The figure shows three views and two pictorial views of one solid part (mm, origin at its lowest corner). Answer the questions. A direction names the side the tool comes from. Round coordinates to 2 decimals unless told otherwise and drop trailing zeros. Order: outer loops, then holes, each group sorted by start corner. A loop starts at its lowest first (then second) coordinate and runs counter-clockwise, first axis right, second up. Notation, with made-up numbers: (85, 38.5) -> (116, 38.5) arc R17 cw to (116, 51.5) -> close; hole circle Ø6 at (80, 78.5). An arc over 180 degrees is marked (long way). Answer as a JSON object with one key per item and string values. Group by question number.
Item 1: Section B-B, the plane z = 38.1 is taken. Write down the section's boundary in (x, y).
Item 2: Section C-C, the plane y = 58.5 is taken. Write down the section's boundary in (x, z), plus the area to 3 significant figures.
Item 3: Consider probe 1 along Y at (x, z) = (6.25, 38.1); probe 2 along Z at (x, y) = (7, 38.1); probe 3 along Z at (x, y) = (11.25, 42.5) (1 decimal). Determine where each line is inside the solid, lowest interval first. Write a range as from..to.
Item 4: Section D-D, the plane z = 68.5 is taken. Write down the section's boundary in (x, y).
Item 5: For the marked faces 1 and 2, determine the directions among +Z, -Z, +X, -X, +Y, -Y from which every point of the face is accessible in a straight line to the end or side of a thin tool.
Item 6: Given P1, Ø3, axis at x = 4.5, y = 91, coming from the -Z side; P2, Ø2.5, axis at x = 8, y = 60.5, coming from the -Z side (1 decimal); P3, Ø4, axis at x = 10, z = 19.5, coming from the +Y side (1 decimal), each flat-ended and moving along its own axis, determine where each tip first touches the part or whether it passes through.
Item 7: The mould has two halves that part along Y. Classify the marked faces 3, 4 and 5: pulls with the +Y half, pulls with the -Y half, needs draft (parallel to the pull), parting line crosses it, or undercut.
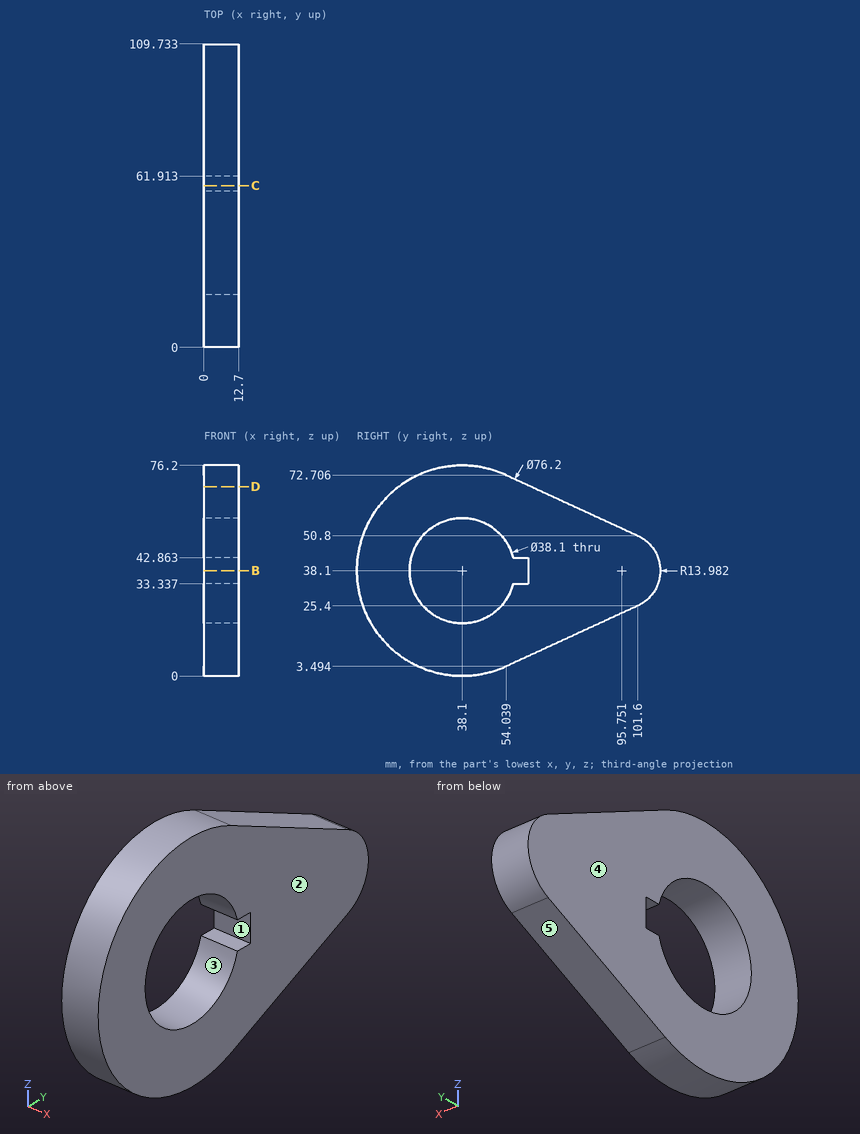
Values found:
{
 "1": {"outline": "(0, 0) -> (12.7, 0) -> (12.7, 19.05) -> (0, 19.05) -> close; (0, 61.91) -> (12.7, 61.91) -> (12.7, 109.73) -> (0, 109.73) -> close"},
 "2": {"outline": "(0, 5.55) -> (12.7, 5.55) -> (12.7, 33.34) -> (0, 33.34) -> close; (0, 42.86) -> (12.7, 42.86) -> (12.7, 70.65) -> (0, 70.65) -> close", "area": "706 mm2"},
 "3": {"probe 1": "0..19.05, 61.91..109.73", "probe 2": "0..19.05, 57.15..76.2", "probe 3": "0.3..19.6, 56.6..75.9"},
 "4": {"outline": "(0, 15.13) -> (12.7, 15.13) -> (12.7, 63.17) -> (0, 63.17) -> close"},
 "5": {"face 1": "+X, -X", "face 2": "+Z, -Z, +X, +Y, -Y"},
 "6": {"P1": "z = 19.83", "P2": "z = 5.9", "P3": "y = 93.1"},
 "7": {"face 3": "undercut", "face 4": "needs draft", "face 5": "pulls with the +Y half"}
}
